Autodesk Inventor part; units mm, degrees
ref_plane "YZ Plane" through (0, 0, 0) normal (1, 0, 0) x (0, 1, 0)
ref_plane "XZ Plane" through (0, 0, 0) normal (0, 1, 0) x (-1, 0, 0)
ref_plane "XY Plane" through (0, 0, 0) normal (0, 0, 1) x (1, 0, 0)
sketch "Sketch1" plane through (0, 0, 0) normal (0, 0, 1) x (1, 0, 0)
  line L0 (-12.2, -17.05) -> (12.2, -17.05)
  line L1 (12.2, -17.05) -> (12.2, 17.05)
  line L2 (12.2, 17.05) -> (-12.2, 17.05)
  line L3 (-12.2, 17.05) -> (-12.2, -17.05)
  line L4 (-12.2, -17.05) -> (12.2, 17.05) construction
  line L5 (12.2, -17.05) -> (-12.2, 17.05) construction
  circle A0 centre (-10, 14.92) radius 1.5
  circle A1 centre (10, 14.92) radius 1.5
  line L6 (-10, 14.92) -> (10, 14.92) construction
  circle A2 centre (-9, 9.05) radius 0.8
  circle A3 centre (-10, 9.05) radius 0.8
  circle A4 centre (9, 9.05) radius 0.8
  circle A5 centre (10, 9.05) radius 0.8
  line L7 (-9, 9.05) -> (9, 9.05) construction
  line L8 (-10, 9.05) -> (10, 9.05) construction
  point P0 (0, 0)
  point P1 (0, 9.05)
  point P2 (0, 14.92)
  point P3 (0, 0)
  point P4 (0, 0)
  dimension "d0" = 24.4
  dimension "d1" = 34.1
  dimension "d2" = 2.13
  dimension "d3" = 3
  dimension "d4" = 10
  dimension "d13" = 20
  dimension "d14" = 18
  dimension "d15" = 1.6
  dimension "d16" = 8
extrude "Extrusion1" add sketch "Sketch1" along normal mid plane 1.6
sketch "Sketch2" plane through (0, 0, -0.8) normal (0, 0, -1) x (-1, 0, 0)
  circle A0 centre (-10, 14.92) radius 1.5
  circle A1 centre (10, 14.92) radius 1.5
  line L0 (-12.2, -17.05) -> (12.2, -17.05)
  line L1 (12.2, -17.05) -> (12.2, 17.05)
  line L2 (12.2, 17.05) -> (-12.2, 17.05)
  line L3 (-12.2, 17.05) -> (-12.2, -17.05)
  line L4 (-10.16, -12.99) -> (10.16, -12.99)
  line L5 (10.16, -12.99) -> (10.16, -15.53)
  line L6 (10.16, -15.53) -> (-10.16, -15.53)
  line L7 (-10.16, -15.53) -> (-10.16, -12.99)
  point P0 (0, 0)
  point P1 (0, -12.99)
  point P2 (-10.16, -14.26)
  dimension "d8" = 2.54
  dimension "d9" = 20.32
  dimension "d10" = 2.79
extrude "Extrusion2" add sketch "Sketch2" along normal blind 2.5 contours L4 L5 L6 L7
sketch "Sketch3" plane through (0, 0, 0.8) normal (0, 0, 1) x (1, 0, 0)
  circle A0 centre (10, 14.92) radius 1.5
  circle A1 centre (-10, 14.92) radius 1.5
  arc A2 (-9.5, 8.4255) -> (-9.5, 9.6745) centre (-9, 9.05) ccw
  arc A3 (-9.5, 9.6745) -> (-9.5, 8.4255) centre (-10, 9.05) ccw
  line L0 (-12.2, -17.05) -> (12.2, -17.05)
  line L1 (12.2, -17.05) -> (12.2, 17.05)
  line L2 (12.2, 17.05) -> (-12.2, 17.05)
  line L3 (-12.2, 17.05) -> (-12.2, -17.05)
  arc A4 (9.5, 9.6745) -> (9.5, 8.4255) centre (9, 9.05) ccw
  arc A5 (9.5, 8.4255) -> (9.5, 9.6745) centre (10, 9.05) ccw
  line L4 (-3.4725, 12.5225) -> (3.4725, 12.5225)
  line L5 (3.4725, 12.5225) -> (3.4725, 5.5775)
  line L6 (3.4725, 5.5775) -> (-3.4725, 5.5775)
  line L7 (-3.4725, 5.5775) -> (-3.4725, 12.5225)
  point P0 (0, 0)
  point P1 (3.4725, 9.05)
  point P2 (0, 12.5225)
  dimension "d17" = 6.945
extrude "Extrusion3" add sketch "Sketch3" along normal blind 0.78 contours L4 L5 L6 L7
sketch "Sketch4" plane through (0, 0, 1.58) normal (0, 0, 1) x (1, 0, 0)
  line L0 (3.4725, 12.5225) -> (-3.4725, 12.5225)
  line L1 (-3.4725, 12.5225) -> (-3.4725, 5.5775)
  line L2 (-3.4725, 5.5775) -> (3.4725, 5.5775)
  line L3 (3.4725, 5.5775) -> (3.4725, 12.5225)
  circle A0 centre (0, 9.05) radius 3.175
  point P0 (0, 0)
  point P1 (0, 12.5225)
  point P2 (-3.4725, 9.05)
  dimension "d20" = 6.35
extrude "Extrusion4" cut sketch "Sketch4" against normal blind 0.1 contours A0
sketch "Sketch5" plane through (0, 0, 0.8) normal (0, 0, 1) x (1, 0, 0)
  line L0 (3.4725, 12.5225) -> (3.4725, 5.5775)
  line L1 (3.4725, 5.5775) -> (-3.4725, 5.5775)
  line L2 (-3.4725, 5.5775) -> (-3.4725, 12.5225)
  line L3 (-3.4725, 12.5225) -> (3.4725, 12.5225)
  circle A0 centre (10, 14.92) radius 1.5
  circle A1 centre (-10, 14.92) radius 1.5
  arc A2 (-9.5, 8.4255) -> (-9.5, 9.6745) centre (-9, 9.05) ccw
  arc A3 (-9.5, 9.6745) -> (-9.5, 8.4255) centre (-10, 9.05) ccw
  line L4 (-12.2, -17.05) -> (12.2, -17.05)
  line L5 (12.2, -17.05) -> (12.2, 17.05)
  line L6 (12.2, 17.05) -> (-12.2, 17.05)
  line L7 (-12.2, 17.05) -> (-12.2, -17.05)
  arc A4 (9.5, 9.6745) -> (9.5, 8.4255) centre (9, 9.05) ccw
  arc A5 (9.5, 8.4255) -> (9.5, 9.6745) centre (10, 9.05) ccw
  line L8 (-11.11, -0.89) -> (11.11, -0.89)
  line L9 (11.11, -0.89) -> (11.11, -11.05)
  line L10 (11.11, -11.05) -> (-11.11, -11.05)
  line L11 (-11.11, -11.05) -> (-11.11, -0.89)
  circle A6 centre (0, 9.05) radius 3.175
  line L12 (0, 1.05) -> (0, -12.99)
  point P0 (0, 0)
  point P1 (0, -0.89)
  point P2 (-11.11, -5.97)
  point P3 (0, -5.97)
  dimension "d24" = 22.22
  dimension "d25" = 10.16
  dimension "d26" = 8
extrude "Extrusion5" add sketch "Sketch5" along normal blind 1.2 contours L8 L12 L10 L11 | L8 L9 L10 L12
sketch "Sketch6" plane through (0, 0, 0.8) normal (0, 0, 1) x (1, 0, 0)
  line L0 (11.11, -0.89) -> (11.11, -11.05)
  line L1 (11.11, -11.05) -> (-11.11, -11.05)
  line L2 (-11.11, -11.05) -> (-11.11, -0.89)
  line L3 (-11.11, -0.89) -> (11.11, -0.89)
  line L4 (3.4725, 12.5225) -> (3.4725, 5.5775)
  line L5 (3.4725, 5.5775) -> (-3.4725, 5.5775)
  line L6 (-3.4725, 5.5775) -> (-3.4725, 12.5225)
  line L7 (-3.4725, 12.5225) -> (3.4725, 12.5225)
  circle A0 centre (10, 14.92) radius 1.5
  circle A1 centre (-10, 14.92) radius 1.5
  arc A2 (-9.5, 8.4255) -> (-9.5, 9.6745) centre (-9, 9.05) ccw
  arc A3 (-9.5, 9.6745) -> (-9.5, 8.4255) centre (-10, 9.05) ccw
  line L8 (-12.2, -17.05) -> (12.2, -17.05)
  line L9 (12.2, -17.05) -> (12.2, 17.05)
  line L10 (12.2, 17.05) -> (-12.2, 17.05)
  line L11 (-12.2, 17.05) -> (-12.2, -17.05)
  arc A4 (9.5, 9.6745) -> (9.5, 8.4255) centre (9, 9.05) ccw
  arc A5 (9.5, 8.4255) -> (9.5, 9.6745) centre (10, 9.05) ccw
  line L12 (11.5, 6.05) -> (9, 6.05)
  line L13 (9, 6.05) -> (9, 2.05)
  line L14 (9, 2.05) -> (11.5, 2.05)
  line L15 (11.5, 2.05) -> (11.5, 6.05)
  line L16 (12.2, 17.05) -> (-12.2, 17.05) construction
  line L17 (-8, 1.05) -> (8, 1.05) construction
  line L18 (8, 1.05) -> (8, 17.05) construction
  line L19 (8, 17.05) -> (-8, 17.05) construction
  line L20 (-8, 17.05) -> (-8, 1.05) construction
  line L21 (-8, 1.05) -> (8, 17.05) construction
  line L22 (8, 1.05) -> (-8, 17.05) construction
  circle A6 centre (0, 9.05) radius 3.175 construction
  point P0 (0, 0)
  dimension "d29" = 2.5
  dimension "d30" = 4
  dimension "d31" = 3
  dimension "d32" = 9
extrude "Extrusion6" add sketch "Sketch6" along normal blind 1.2 contours L15 L14 L13 L12
sketch "Sketch7" plane through (0, 0, -0.8) normal (0, 0, -1) x (-1, 0, 0)
  line L0 (6, -8) -> (-6, -8)
  line L1 (-6, -8) -> (-6, 4)
  line L2 (-6, 4) -> (6, 4)
  line L3 (6, 4) -> (6, -8)
  line L4 (6, -8) -> (-6, 4) construction
  line L5 (-6, -8) -> (6, 4) construction
  point P0 (0, 0)
  point P1 (0, -2)
  point P2 (0, -2)
  dimension "d35" = 12
  dimension "d36" = 2
extrude "Extrusion7" add sketch "Sketch7" along normal blind 1.2
fillet "Fillet1" radius 0.5 4 edges at (9, 6.05, 1.4) (11.5, 6.05, 1.4) (11.5, 2.05, 1.4) (9, 2.05, 1.4)
equation "\"d9\" = 8 * d8"
properties part number "66-0005" material "Epoxy Resin"
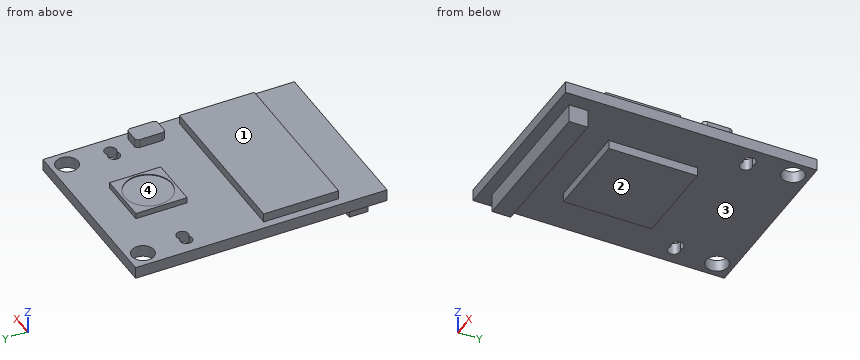
Could you check a few things on this model? Use its own coordinates, in mm. Face numbers are marked on the shaded views. A direction names the side the tool comes from. Round coordinates to 2 decimals unless told otherwise and drop trailing zeros. Loops run counter-clockwise (first coordinate to the right, second up) from the corner with the lowest first, then second, coordinate; pieces in that order, holes last. Notation, with made-up numbers: (-16, -1) -> (-7, -1) arc R11 cw to (-7, 9) -> close; hole circle Ø3 at (29, 86.25). An arc over 180 degrees is marked (long way). Put each result on its own line as item: value.
Q1. Thinking about a two-plate mould opening in X: for the marked faces 3 and 4, which applies, pulls with the +X half, pulls with the -X half, needs draft (parallel to the pull), parting line crosses it, or undercut?
Checks:
face 3: needs draft
face 4: undercut
Q2. For pin 1 Ø0.9 at (y, z) = (8.5, 1.5) entering from +X; pin 2 Ø3 at (x, y) = (0.5, 8.5) entering from +Z; pin 3 Ø1.5 at (x, z) = (0.5, -2.5) entering from +Y; pin 4 Ø1 at (y, z) = (5.5, -3) entering from -X, each with a flat end and sliding along its axis, tell me the tip position at first contact or that it passes through.
Checks:
pin 1: x = 3.47
pin 2: z = 1.48
pin 3: y = 4
pin 4: through
Q3. Which directions (+Z, -Z, +X, -X, +Y, -Y) give clear straight access to the entire face, cutting with the end or side of a thin tool? Please do the marked faces 1 and 2.
Checks:
face 1: +Z, +X, -X, +Y, -Y
face 2: -Z, +X, -X, +Y
Q4. Please list where these lines run through material, in increasing order: line 1 (Y direction, x = 10, z = 0.35); line 2 (Y direction, x = -4.5, z = -0.85); line 3 (Y direction, x = -8.75, z = -0.25). Write a range as from..to.
Checks:
line 1: -17.05..8.25, 9.85..13.42, 16.42..17.05
line 2: -15.53..-12.99, -8..4
line 3: -17.05..8.29, 9.81..14.09, 15.75..17.05
Q5. I want a section at A-A on y = 9.05. Give the number of separate pieces and of enclosed holes in the cut face, and give its area (3 significant figures).
Checks:
separate pieces: 3
enclosed holes: 0
area: 35.5 mm2
Q6. I want a section at B-B on x = -4. Write out the boundary of the cut face in (y, z), and give its area (3 significant figures).
Checks:
outline: (-17.05, -0.8) -> (-15.53, -0.8) -> (-15.53, -3.3) -> (-12.99, -3.3) -> (-12.99, -0.8) -> (-8, -0.8) -> (-8, -2) -> (4, -2) -> (4, -0.8) -> (17.05, -0.8) -> (17.05, 0.8) -> (-0.89, 0.8) -> (-0.89, 2) -> (-11.05, 2) -> (-11.05, 0.8) -> (-17.05, 0.8) -> close
area: 87.5 mm2
Q7. I want a section at C-C on y = -3.5. Write out the boundary of the cut face in (x, z).
Checks:
outline: (-12.2, -0.8) -> (-6, -0.8) -> (-6, -2) -> (6, -2) -> (6, -0.8) -> (12.2, -0.8) -> (12.2, 0.8) -> (11.11, 0.8) -> (11.11, 2) -> (-11.11, 2) -> (-11.11, 0.8) -> (-12.2, 0.8) -> close
Q8. I want a section at D-D on x = -9. Write out the boundary of the cut face in (y, z), and give its area (3 significant figures).
Checks:
outline: (-17.05, -0.8) -> (-15.53, -0.8) -> (-15.53, -3.3) -> (-12.99, -3.3) -> (-12.99, -0.8) -> (8.25, -0.8) -> (8.25, 0.8) -> (-0.89, 0.8) -> (-0.89, 2) -> (-11.05, 2) -> (-11.05, 0.8) -> (-17.05, 0.8) -> close; (9.85, -0.8) -> (13.8, -0.8) -> (13.8, 0.8) -> (9.85, 0.8) -> close; (16.04, -0.8) -> (17.05, -0.8) -> (17.05, 0.8) -> (16.04, 0.8) -> close
area: 67.0 mm2
